Here's how the part is built. I have some questions about the finished solid (model axes, mm). Face numbers are marked on the shaded views. A direction names the side the tool comes from. Round coordinates to 2 decimals unless told otherwise and drop trailing zeros. Loops run counter-clockwise (first coordinate to the right, second up) from the corner with the lowest first, then second, coordinate; pieces in that order, holes last. Notation, with made-up numbers: (66, -32.75) -> (117, -32.75) arc R32 ccw to (117, 5.25) -> close; hole circle Ø3 at (18, 58.25). An arc over 180 degrees is marked (long way). One line per item, written item: value. Start each with the question number.
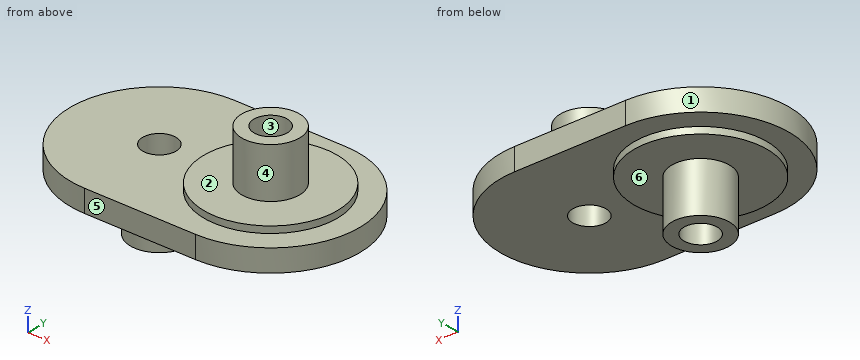
```python
from build123d import *

# Parameters (mm, degrees)
CYLINDER009_R     = 1.5
CYLINDER009_DEPTH = 7.1
CYLINDER007_R     = 1.5
CYLINDER007_DEPTH = 7.1
CYLINDER006_R     = 6
CYLINDER006_DEPTH = 2.6
CYLINDER008_R     = 2.6
CYLINDER008_DEPTH = 7.1
CYLINDER010_R     = 2.6
CYLINDER010_DEPTH = 7.1
PAD_DEPTH         = 2
CYLINDER005_R     = 6
CYLINDER005_DEPTH = 2.6


with BuildPart() as cylinder009:
    # Cylinder009 → Cylinder009 (new body)
    with BuildSketch(Plane(origin=(-5, 0, -5.1), x_dir=(1, 0, 0), z_dir=(0, 0, 1))):
        Circle(CYLINDER009_R)
    extrude(amount=CYLINDER009_DEPTH)


with BuildPart() as idle_linkage_hole_fusion:
    # Cylinder007 → Cylinder007 (new body)
    with BuildSketch(Plane(origin=(5, 0, 0), x_dir=(1, 0, 0), z_dir=(0, 0, 1))):
        Circle(CYLINDER007_R)
    extrude(amount=CYLINDER007_DEPTH)

    # Fusion009: union Cylinder009
    add(cylinder009.part)


with BuildPart() as cylinder006:
    # Cylinder006 → Cylinder006 (new body)
    with BuildSketch(Plane(origin=(-5, 0, -0.6), x_dir=(1, 0, 0), z_dir=(0, 0, 1))):
        Circle(CYLINDER006_R)
    extrude(amount=CYLINDER006_DEPTH)


with BuildPart() as cylinder008:
    # Cylinder008 → Cylinder008 (new body)
    with BuildSketch(Plane(origin=(5, 0, 0), x_dir=(1, 0, 0), z_dir=(0, 0, 1))):
        Circle(CYLINDER008_R)
    extrude(amount=CYLINDER008_DEPTH)


with BuildPart() as cylinder010:
    # Cylinder010 → Cylinder010 (new body)
    with BuildSketch(Plane(origin=(-5, 0, -5.1), x_dir=(1, 0, 0), z_dir=(0, 0, 1))):
        Circle(CYLINDER010_R)
    extrude(amount=CYLINDER010_DEPTH)


with BuildPart() as idle_linkage_base_body:
    # Sketch008 → Pad (new body)
    with BuildSketch(Plane.XY):
        with BuildLine():
            Line((-5, 8), (5, 8))
            ThreePointArc((5, -8), (13, 0), (5, 8))
            Line((-5, -8), (5, -8))
            ThreePointArc((-5, 8), (-13, 0), (-5, -8))
        make_face()
    extrude(amount=PAD_DEPTH)


with BuildPart() as idle_fusion_cut:
    # Cylinder005 → Cylinder005 (new body)
    with BuildSketch(Plane(origin=(5, 0, 0), x_dir=(1, 0, 0), z_dir=(0, 0, 1))):
        Circle(CYLINDER005_R)
    extrude(amount=CYLINDER005_DEPTH)

    # Fusion008: union Cylinder006, Cylinder008, Cylinder010, idle linkage base body
    add(cylinder006.part)
    add(cylinder008.part)
    add(cylinder010.part)
    add(idle_linkage_base_body.part)

    # Cut001: cut idle linkage hole fusion
    add(idle_linkage_hole_fusion.part, mode=Mode.SUBTRACT)


solid = idle_fusion_cut.part
```
Q1. Which directions (+Z, -Z, +X, -X, +Y, -Y) give clear straight access to the entire face, cutting with the end or side of a thin tool? Please do the marked faces 4, 5 and 6.
Q2. If I drill on line 1 along Y through (x, z) = (5, 5.75); line 2 along Z through (x, y) = (5.5, -7); line 3 along Z through (x, y) = (8.75, -2.25), over which ranges is the centre line in solid material (lowest first)?
Q3. Will these pins go through, and if not, where does the flat tip stop? P1, Ø3, axis at x = -0.5, z = -1, coming from the +Y side; P2, Ø5, axis at x = 1, y = -4, coming from the +Z side; P3, Ø2.5, axis at x = 5, y = 0, coming from the -Z side; P4, Ø1.5, axis at x = 5, z = 4.5, coming from the -Y side.
Q4. I want a section at A-A on y = 0. Please give me the cut outline in (x, z), plus the area to 3 significant figures.
Q5. I want a section at C-C on x = 4. Please give me the cut outline in (y, z).
Q6. If we mould it in two halves opening along X, with no side actions, what happens to the marked faces 1, 2 and 3? For each: released by +X, released by -X, zero draft, split by the parting line, or undercut.
Q7. I want a section at D-D on y = 4.25. Please give me the cut outline in (x, z), plus the area to 3 significant figures.
Q8. I want a section at B-B on z = 1. Please give me the cut outline in (x, y).
Answers below:
1. face 4: +Z
1. face 5: +Z, -Z, +X, -X, -Y
1. face 6: -Z
2. line 1: y = -2.6 to -1.5, 1.5 to 2.6
2. line 2: z = 0 to 2
2. line 3: z = 0 to 2.6
3. P1: stops at y = 8
3. P2: stops at z = 2.6
3. P3: passes through
3. P4: stops at y = -2.6
4. outline: (-13, 0) -> (-11, 0) -> (-11, -0.6) -> (-7.6, -0.6) -> (-7.6, -5.1) -> (-6.5, -5.1) -> (-6.5, 2) -> (-13, 2) -> close; (-3.5, -5.1) -> (-2.4, -5.1) -> (-2.4, -0.6) -> (1, -0.6) -> (1, 0) -> (3.5, 0) -> (3.5, 7.1) -> (2.4, 7.1) -> (2.4, 2.6) -> (-1, 2.6) -> (-1, 2) -> (-3.5, 2) -> close; (6.5, 0) -> (13, 0) -> (13, 2) -> (11, 2) -> (11, 2.6) -> (7.6, 2.6) -> (7.6, 7.1) -> (6.5, 7.1) -> close
4. area: 70.6 mm^2
5. outline: (-8, 0) -> (-1.12, 0) -> (-1.12, 7.1) -> (-2.4, 7.1) -> (-2.4, 2.6) -> (-5.92, 2.6) -> (-5.92, 2) -> (-8, 2) -> close; (1.12, 0) -> (8, 0) -> (8, 2) -> (5.92, 2) -> (5.92, 2.6) -> (2.4, 2.6) -> (2.4, 7.1) -> (1.12, 7.1) -> close
6. face 1: released by -X
6. face 2: zero draft
6. face 3: undercut
7. outline: (-11.78, 0) -> (-9.24, 0) -> (-9.24, -0.6) -> (-0.76, -0.6) -> (-0.76, 0) -> (11.78, 0) -> (11.78, 2) -> (9.24, 2) -> (9.24, 2.6) -> (0.76, 2.6) -> (0.76, 2) -> (-11.78, 2) -> close
7. area: 57.3 mm^2
8. outline: (-5, -8) -> (5, -8) arc R8 ccw to (5, 8) -> (-5, 8) arc R8 ccw to start; hole circle Ø3 at (-5, 0); hole circle Ø3 at (5, 0)
